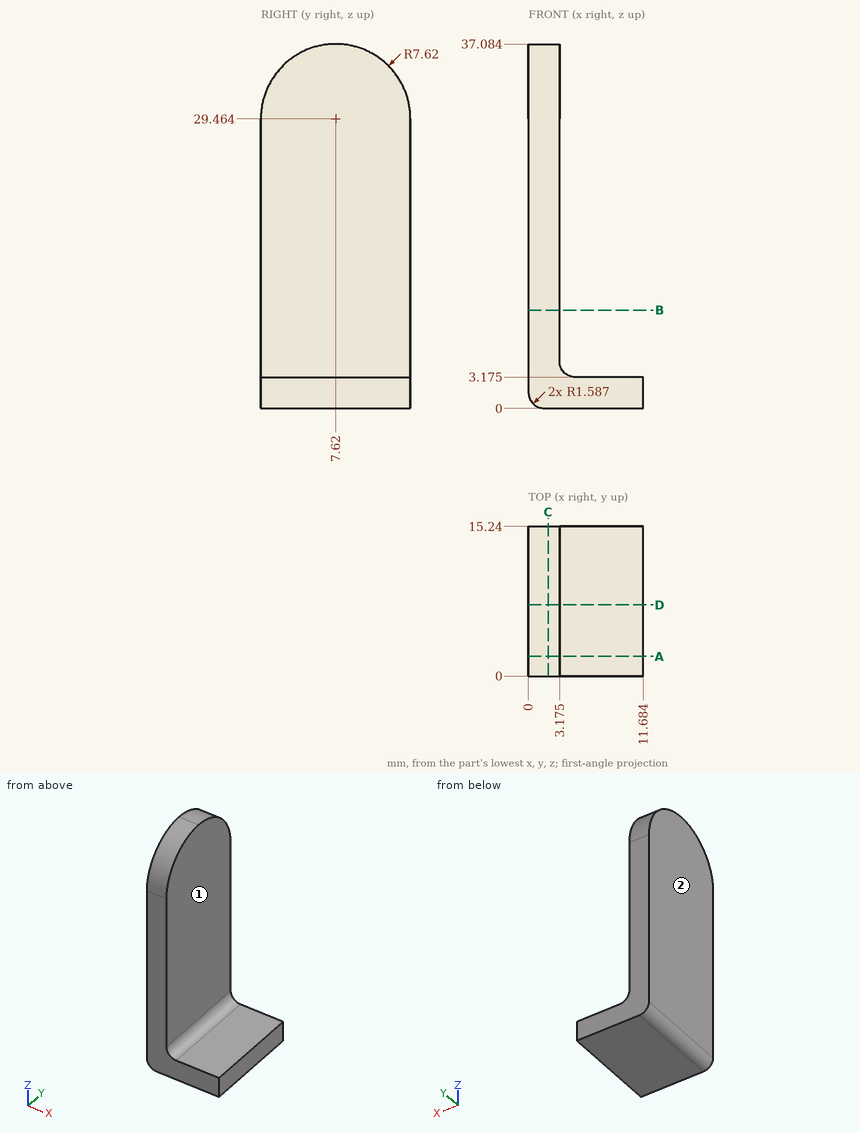
The drawing under review shows one solid part. Ordinate dimensions are in mm from its lowest x, y, z. A direction names the side the tool comes from. Coordinates: 2 decimals unless noted, no trailing zeros. Order: outer loops, then holes, each group sorted by start corner. A loop starts at its lowest first (then second) coordinate and runs counter-clockwise, first axis right, second up. Notation, with made-up numbers: (-26, 30.5) -> (-19, 30.5) arc R15 cw to (-19, 54.5) -> close; hole circle Ø5 at (84.5, -17). An arc over 180 degrees is marked (long way). Use CSV: the item, a comma, the result in double quotes. Start each with the question number.
Item 1: We need section A-A, the plane y = 2. Give the boundary of the cut face in (x, z) (1 decimal).
Item 2: We need section C-C, the plane x = 2. Give the boundary of the cut face in (y, z) (1 decimal).
Item 3: We need section B-B, the plane z = 10. Give the boundary of the cut face in (x, y) (1 decimal).
Item 4: We need section D-D, the plane y = 7.25. Give the boundary of the cut face in (x, z) (1 decimal), then the cut area to 3 significant figures.
Item 5: Insertion check: pin 1 (6 mm diameter, centred on x = 7, y = 5, fed in from +Z); pin 2 (5.5 mm diameter, centred on x = 9, y = 9, fed in from +Z) (1 decimal). Each pin has a flat end and moves straight along its axis. Give the tip position at first contact, or say it passes through.
Item 6: For the marked faces 1 and 2, list the 3-axis set-ups (+Z, -Z, +X, -X, +Y, -Y) from which the entire face can be reached by the end or side of a thin tool; tool diameter is ignored.
Item 7: Wall thickness on probe 1 along Z at (x, y) = (9.25, 8.25) (1 decimal); probe 2 along Z at (x, y) = (3, 12.75): over which ranges is each line inside the solid? List them lowest first.
Derived:
1,outline,"(0, 1.6) arc R1.6 ccw to (1.6, 0) -> (11.7, 0) -> (11.7, 3.2) -> (4.8, 3.2) arc R1.6 cw to (3.2, 4.8) -> (3.2, 34.6) -> (0, 34.6) -> close"
2,outline,"(0, 0) -> (15.2, 0) -> (15.2, 29.5) arc R7.6 ccw to (0, 29.5) -> close"
3,outline,"(0, 0) -> (3.2, 0) -> (3.2, 15.2) -> (0, 15.2) -> close"
4,outline,"(0, 1.6) arc R1.6 ccw to (1.6, 0) -> (11.7, 0) -> (11.7, 3.2) -> (4.8, 3.2) arc R1.6 cw to (3.2, 4.8) -> (3.2, 37.1) -> (0, 37.1) -> close"
4,area,"145 mm^2"
5,pin 1,"stops at z = 3.37"
5,pin 2,"stops at z = 3.2"
6,face 1,"+Z, +X, +Y, -Y"
6,face 2,"+Z, -Z, -X, +Y, -Y"
7,probe 1,"z = 0 to 3.2"
7,probe 2,"z = 0 to 35.1"
